```python
from build123d import *

# Parameters (mm, degrees)
SKETCH1_R           = 5.5626
BOSS_EXTRUDE1_DEPTH = 4.7625
SKETCH2_R           = 3.96875
BOSS_EXTRUDE2_DEPTH = 7.9375
SKETCH3_R           = 1.5875
CUT_EXTRUDE1_DEPTH  = 15.939044063
CHAMFER1_SIZE       = 0.254


with BuildPart() as part:
    # Sketch1 → Boss-Extrude1 (new body)
    with BuildSketch(Plane.XY):
        with Locations(Location((0, 0, 0), (0, 0, 180))):
            Circle(SKETCH1_R)
    extrude(amount=BOSS_EXTRUDE1_DEPTH)

    # Sketch2 → Boss-Extrude2 (add)
    with BuildSketch(Plane.XY.offset(4.7625)):
        Circle(SKETCH2_R)
    extrude(amount=BOSS_EXTRUDE2_DEPTH)

    # Sketch3 → Cut-Extrude1 (cut, through all)
    with BuildSketch(Plane(origin=(0, 0, 0), x_dir=(-1, 0, 0), z_dir=(0, 0, -1))):
        Circle(SKETCH3_R)
    extrude(amount=-CUT_EXTRUDE1_DEPTH, mode=Mode.SUBTRACT)

    # Chamfer1
    chamfer1_edges = [part.edges().sort_by_distance(p)[0] for p in [
        (1.5875, 0, 12.7),
        (1.5875, 0, 0),
        (-3.96875, 0, 12.7),
    ]]
    chamfer(chamfer1_edges, length=CHAMFER1_SIZE)


solid = part.part
```
Design review of the part built by this model. Coordinates are the model's own, in mm. A direction names the side the tool comes from. Round coordinates to 2 decimals unless told otherwise and drop trailing zeros. Write each loop counter-clockwise with the first axis right and the second up, starting at its lowest first coordinate (ties: lowest second). Pieces come first, ordered by that corner, then holes.
Item 1: Clearance check with flat-ended pins moving along their axes: pin 1 Ø4 at (x, y) = (4, -3) entering from +Z; pin 2 Ø2 at (x, z) = (-3.5, 8.5) entering from +Y; pin 3 Ø5 at (y, z) = (-4, 10) entering from -X; pin 4 Ø2 at (y, z) = (3.5, 8.5) entering from +X. State where each tip first meets the part, or that it passes through.
Item 2: For faces 4 (the flat face through (1, -4, 4.762)), 5 (the cylindrical face through (-5.306, -1.671, 2.348)), list the 3-axis set-ups (+Z, -Z, +X, -X, +Y, -Y) from which the entire face can be reached by the end or side of a thin tool; tool diameter is ignored.
Item 3: We need section D-D on y = -4.25. Write out the cut boundary in (x, z).
Item 4: We need section A-A on y = 0. Write out the cut boundary in (x, z).
Item 5: We need section C-C on z = 1.5. Write out the cut boundary in (x, y) (1 decimal), and give its area (3 significant figures).
Item 6: The part is to be moulded in two halves that separate along Y. For faces 1 (the flat face through (-2, -1, 12.7)), 2 (the cylindrical face through (-0.86, -3.874, 8.55)), 3 (the cylindrical face through (0.34, -1.55, 6.26)), say which applies: +Y half, -Y half, draft (parallel to the pull), parting line (faces both ways), or undercut.
Item 7: For probe 1 along Y at (x, z) = (0, 9.5); probe 2 along Z at (x, y) = (2.75, 4.25); probe 3 along X at (y, z) = (0.75, 2), list the stretches that pass through material, from the lowest coordinate up.
Returned:
1. pin 1: stops at z = 12.7
1. pin 2: stops at y = 3.08
1. pin 3: stops at x = -3.67
1. pin 4: stops at x = 3.08
2. face 4: +Z
2. face 5: +Z, -Z
3. outline: (-3.59, 0) - (3.59, 0) - (3.59, 4.76) - (-3.59, 4.76) - close
4. outline: (-5.56, 0) - (-1.84, 0) - (-1.59, 0.25) - (-1.59, 12.45) - (-1.84, 12.7) - (-3.71, 12.7) - (-3.97, 12.45) - (-3.97, 4.76) - (-5.56, 4.76) - close; (1.59, 0.25) - (1.84, 0) - (5.56, 0) - (5.56, 4.76) - (3.97, 4.76) - (3.97, 12.45) - (3.71, 12.7) - (1.84, 12.7) - (1.59, 12.45) - close
5. outline: circle Ø11.1 at (0, 0); hole circle Ø3.2 at (0, 0)
5. area: 89.3 mm2
6. face 1: draft
6. face 2: parting line
6. face 3: undercut
7. probe 1: y = -3.97 to -1.59, 1.59 to 3.97
7. probe 2: z = 0 to 4.76
7. probe 3: x = -5.51 to -1.4, 1.4 to 5.51
